Could you check a few things on this drawing? It's one solid part, dimensions in mm from its lowest x, y, z. A direction names the side the tool comes from. Give positions to 0.01 mm unless a question says otherwise; leave off trailing zeros. Order: outer loops, then holes, each group sorted by start corner. A loop starts at its lowest first (then second) coordinate and runs counter-clockwise, first axis right, second up. Notation, with made-up numbers: (47, 22.25) - (90, 22.25) arc R27 ccw to (90, 55.25) - close; hole circle Ø10 at (-12.75, 46). An arc over 180 degrees is marked (long way). Put each result on its own line as item: value.
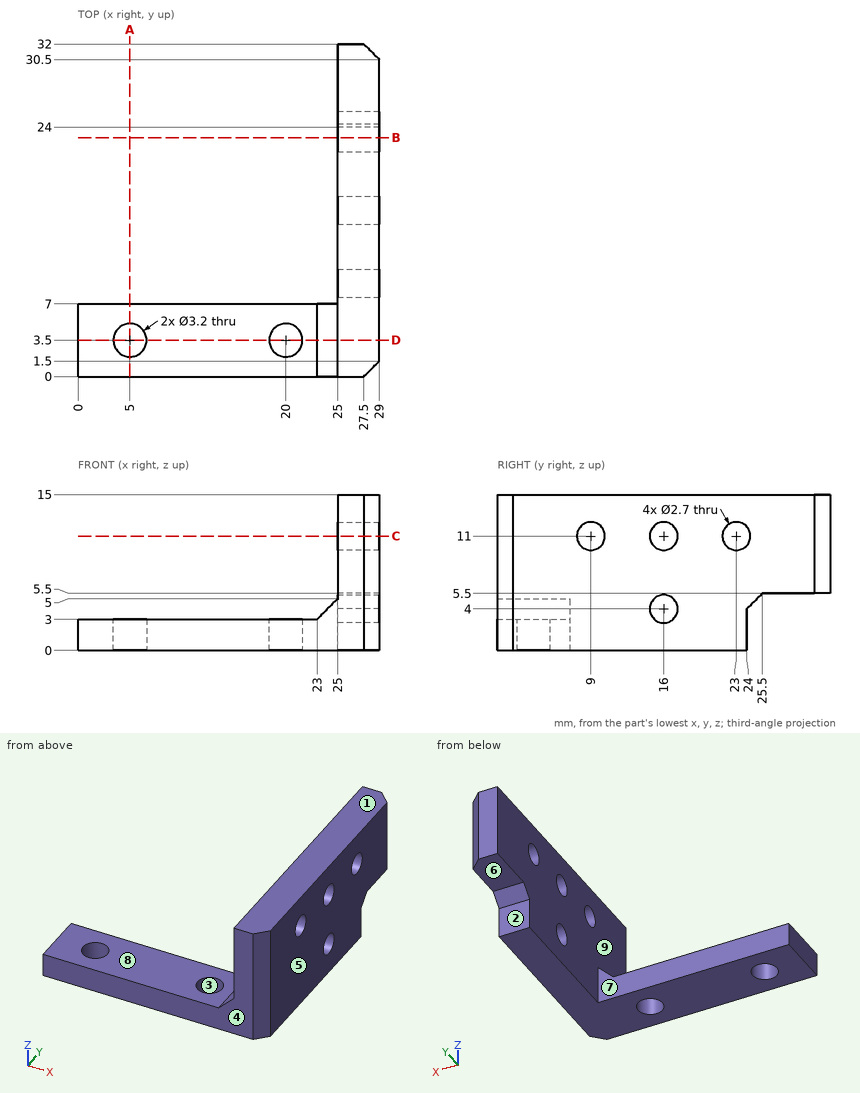
1) Suppose I cut it at D-D, the plane y = 3.5. List the corners of the cut face in (x, z) for me, and give its area (3 significant figures).
Filled in:
outline: (0, 0) - (3.4, 0) - (3.4, 3) - (0, 3) - close; (6.6, 0) - (18.4, 0) - (18.4, 3) - (6.6, 3) - close; (21.6, 0) - (29, 0) - (29, 15) - (25, 15) - (25, 5) - (23, 3) - (21.6, 3) - close
area: 118 mm^2
2) If I drill on line 1 (Y direction, x = 27.3, z = 11); line 2 (Y direction, x = 20, z = 2.25); line 3 (X direction, y = 14, z = 4.75), over which ranges is the centre line in solid material (lowest first)? Write a range as [from, to].
Filled in:
line 1: y = [0, 7.65], [10.35, 14.65], [17.35, 21.65], [24.35, 32]
line 2: y = [0, 1.9], [5.1, 7]
line 3: x = [25, 29]
3) Suppose I cut it at C-C, the plane z = 11. List the corners of the cut face in (x, y) for me.
Filled in:
outline: (25, 0) - (27.5, 0) - (29, 1.5) - (29, 7.65) - (25, 7.65) - close; (25, 10.35) - (29, 10.35) - (29, 14.65) - (25, 14.65) - close; (25, 17.35) - (29, 17.35) - (29, 21.65) - (25, 21.65) - close; (25, 24.35) - (29, 24.35) - (29, 30.5) - (27.5, 32) - (25, 32) - close
4) Suppose I cut it at A-A, the plane x = 5. List the corners of the cut face in (y, z) for me.
Filled in:
outline: (0, 0) - (1.9, 0) - (1.9, 3) - (0, 3) - close; (5.1, 0) - (7, 0) - (7, 3) - (5.1, 3) - close
5) Which directions (+Z, -Z, +X, -X, +Y, -Y) give clear straight access to the entire face, cutting with the end or side of a thin tool? Please do the marked faces 5, 6, 7, 8 and 9.
Filled in:
face 5: +Z, -Z, +X, +Y, -Y
face 6: -Z, +X, -X, +Y
face 7: +Z, -Z, -X, +Y
face 8: +Z, -X, +Y, -Y
face 9: +Z, -X, +Y
6) We'd pull the mould along Y, two halves only. Please class the marked faces 1, 2, 3 and 4: pulls with the +Y half, pulls with the -Y half, needs draft (parallel to the pull), parting line crosses it, or undercut.
Filled in:
face 1: needs draft
face 2: pulls with the +Y half
face 3: undercut
face 4: pulls with the -Y half
7) Suppose I cut it at B-B, the plane y = 23. List the corners of the cut face in (x, z) for me, and give its area (3 significant figures).
Filled in:
outline: (25, 0) - (29, 0) - (29, 9.65) - (25, 9.65) - close; (25, 12.35) - (29, 12.35) - (29, 15) - (25, 15) - close
area: 49.2 mm^2
8) I'm going to push flat-ended pins straight in: pin 1 (7.5 mm diameter, centred on y = 21.5, z = 5.5, fed in from -X); pin 2 (5.5 mm diameter, centred on x = 14, z = 2.5, fed in from +Y); pin 3 (3 mm diameter, centred on x = 27, z = 1, fed in from +Y). Where does each tip first touch, or does it pass through?
Filled in:
pin 1: stops at x = 25
pin 2: stops at y = 7
pin 3: stops at y = 24
